```python
from build123d import *

# Parameters (mm, degrees)
BOSS_EXTRUDE1_DEPTH = 17.5
BOSS_EXTRUDE2_DEPTH = 5
CUT_EXTRUDE1_DEPTH  = 97.89865525603899
CUT_EXTRUDE2_DEPTH  = 97.89865525603899
CUT_EXTRUDE3_DEPTH  = 97.89865525603899
CUT_EXTRUDE4_DEPTH  = 97.89865525603899
CUT_EXTRUDE5_DEPTH  = 97.898655256039
HOLE1_D             = 3.4
HOLE2_D             = 8.4
HOLE3_D             = 4.4
HOLE4_D             = 23
HOLE5_D             = 8.4
HOLE6_D             = 4.4
FILLET1_R           = 8
CHAMFER1_SIZE       = 3.2892742843300167
CHAMFER1_SIZE2      = 5.503472902596259
CHAMFER2_SIZE       = 1.0000000000000073
CHAMFER3_SIZE       = 3.9999999999999973
CHAMFER4_SIZE       = 1.9999999999999982
CHAMFER5_SIZE       = 1.154784669
CHAMFER6_SIZE       = 0.9999999999999983
FILLET2_R           = 5
FILLET3_R           = 8.99999999999999
FILLET4_R           = 9.000000000000002


with BuildPart() as part:
    # Sketch1 → Boss-Extrude1 (new body)
    with BuildSketch(Plane(origin=(0, 0, 0), x_dir=(-6e-17, -1, 0), z_dir=(-1, 6e-17, 0))):
        with BuildLine():
            Line((11.200465877219063, 72.38053808131822), (-8.757531911002138, 37.812271894771776))
            ThreePointArc((-8.757531911002138, 37.812271894771776), (-19.5478712071735, 38.906001767514), (-24.988655696858714, 29.523809523809472))
            Line((-24.988655696858714, 29.523809523809472), (-23.581163303210467, 5.42e-15))
            Line((-23.581163303210467, 5.42e-15), (46.60534104687875, -6.94e-15))
            Line((46.60534104687875, -6.94e-15), (62.00126690227817, 42.299958639307405))
            Line((62.00126690227817, 42.299958639307405), (11.200465877219063, 72.38053808131822))
        make_face()
    extrude(amount=-BOSS_EXTRUDE1_DEPTH)

    # Sketch2 → Boss-Extrude2 (add)
    with BuildSketch(Plane(origin=(0, 0, 0), x_dir=(-6e-17, -1, 0), z_dir=(-1, 6e-17, 0))):
        with BuildLine():
            Line((-8.757531911002138, 37.812271894771776), (3.3020035333110394, 58.69999999999994))
            Line((3.3020035333110394, 58.69999999999994), (-12.000000000000004, 58.699999999999946))
            Line((-12.000000000000004, 58.699999999999946), (-12.000000000000004, 39.539392014169366))
            ThreePointArc((-12.000000000000004, 39.539392014169366), (-10.298772493194686, 38.826010419734104), (-8.757531911002138, 37.812271894771776))
        make_face()
    extrude(amount=-BOSS_EXTRUDE2_DEPTH)

    # Sketch3 → Cut-Extrude1 (cut, through all)
    with BuildSketch(Plane.ZY):
        with BuildLine():
            Line((18.94418997404675, -15.937202057164905), (20.43837116769735, -19.141483967443826))
            ThreePointArc((20.43837116769735, -19.141483967443826), (22.697545450618843, -19.96375616044696), (23.519817643621966, -17.70458187752546))
            Line((23.519817643621966, -17.70458187752546), (22.02563644997135, -14.500299967246516))
            ThreePointArc((22.02563644997135, -14.500299967246516), (19.766462167049855, -13.67802777424341), (18.94418997404675, -15.937202057164905))
        make_face()
    extrude(amount=-CUT_EXTRUDE1_DEPTH, mode=Mode.SUBTRACT)

    # Sketch4 → Cut-Extrude2 (cut, through all)
    with BuildSketch(Plane.ZY):
        with BuildLine():
            Line((48.89693341141304, -24.280652217339153), (45.692651501134065, -25.774833410989757))
            ThreePointArc((45.692651501134065, -25.774833410989757), (44.87037930813095, -28.034007693911235), (47.12955359105242, -28.85627988691438))
            Line((47.12955359105242, -28.85627988691438), (50.33383550133139, -27.362098693263775))
            ThreePointArc((50.33383550133139, -27.362098693263775), (51.156107694334516, -25.102924410342293), (48.89693341141304, -24.280652217339153))
        make_face()
    extrude(amount=-CUT_EXTRUDE2_DEPTH, mode=Mode.SUBTRACT)

    # Sketch5 → Cut-Extrude3 (cut, through all)
    with BuildSketch(Plane.ZY):
        with BuildLine():
            Line((35.97785558166356, -52.46601583434486), (37.47203677531419, -55.6702977446238))
            ThreePointArc((37.47203677531419, -55.6702977446238), (39.73121105823568, -56.4925699376269), (40.55348325123879, -54.233395654705404))
            Line((40.55348325123879, -54.233395654705404), (39.059302057588205, -51.02911374442645))
            ThreePointArc((39.059302057588205, -51.02911374442645), (36.80012777466672, -50.20684155142337), (35.97785558166356, -52.46601583434486))
        make_face()
    extrude(amount=-CUT_EXTRUDE3_DEPTH, mode=Mode.SUBTRACT)

    # Sketch6 → Cut-Extrude4 (cut, through all)
    with BuildSketch(Plane.ZY):
        with BuildLine():
            Line((10.600739813872503, -45.8899454945312), (13.805021724151473, -44.395764300880586))
            ThreePointArc((13.805021724151473, -44.395764300880586), (14.627293917154569, -42.136590017959094), (12.36811963423308, -41.314317824955985))
            Line((12.36811963423308, -41.314317824955985), (9.163837723954103, -42.8084990186066))
            ThreePointArc((9.163837723954103, -42.8084990186066), (8.341565530951023, -45.06767330152808), (10.600739813872503, -45.8899454945312))
        make_face()
    extrude(amount=-CUT_EXTRUDE4_DEPTH, mode=Mode.SUBTRACT)

    # Sketch7 → Cut-Extrude5 (cut, through all)
    with BuildSketch(Plane(origin=(17.5, -1.07e-15, 0), x_dir=(0, 0, -1), z_dir=(1, -6e-17, 0))):
        Polygon((-30.000000000000007, 8.000000000000005), (-30.000000000000007, -9.938112905604582), (-16.55393055212617, -9.938112905604578), (-10.000000000000002, -27.94488910624502), (-10.000000000000002, 8.000000000000005), align=None)
    extrude(amount=-CUT_EXTRUDE5_DEPTH, mode=Mode.SUBTRACT)

    # Hole1 (through all)
    with Locations(Plane(origin=(5, -3.1e-16, 0), x_dir=(0, 0, -1), z_dir=(1, -6e-17, 0))):
        with Locations((-50.7, 7)):
            Hole(HOLE1_D / 2)

    # Hole2 (through all)
    with Locations(Plane.ZY):
        with Locations((9, 15)):
            Hole(HOLE2_D / 2)

    # Hole3 (through all)
    with Locations(Plane.ZY):
        with Locations((40.5, -12.150669091)):
            Hole(HOLE3_D / 2)

    # Hole4 (through all)
    with Locations(Plane.ZY):
        with Locations((29.748836613, -35.085298856)):
            Hole(HOLE4_D / 2)

    # Hole5 (through all)
    with Locations(Plane.ZY):
        with Locations((60, -14.444863729)):
            Hole(HOLE5_D / 2)

    # Hole6 (through all)
    with Locations(Plane.ZY):
        with Locations((30, 15)):
            Hole(HOLE6_D / 2)

    # Fillet1
    fillet1_edges = [part.edges().sort_by_distance(p)[0] for p in [
        (11.25, 8.757531911002138, 37.812271894771776),
    ]]
    fillet(fillet1_edges, radius=FILLET1_R)

    # Chamfer1
    chamfer1_edges = [part.edges().sort_by_distance(p)[0] for p in [
        (8.75, -9.93811290560458, 16.55393055212617),
    ]]
    chamfer1_side = [part.faces().sort_by_distance(p)[0] for p in [
        (8.750000000000002, -18.941501005924803, 13.276965276063088),
    ]]
    chamfer(chamfer1_edges, length=CHAMFER1_SIZE, length2=CHAMFER1_SIZE2, reference=chamfer1_side[0])

    # Chamfer2
    chamfer2_edges = [part.edges().sort_by_distance(p)[0] for p in [
        (2.5, -3.3020035333110394, 58.69999999999994),
    ]]
    chamfer(chamfer2_edges, length=CHAMFER2_SIZE)

    # Chamfer3
    chamfer3_edges = [part.edges().sort_by_distance(p)[0] for p in [
        (2.500000000000001, 12.000000000000004, 58.699999999999946),
    ]]
    chamfer(chamfer3_edges, length=CHAMFER3_SIZE)

    # Chamfer4
    chamfer4_edges = [part.edges().sort_by_distance(p)[0] for p in [
        (8.75, 8.000000000000004, 10.000000000000002),
    ]]
    chamfer(chamfer4_edges, length=CHAMFER4_SIZE)

    # Chamfer5
    # the kernel refuses this chamfer: 1.339656624, 1.154784669 mm, written as the material it adds along each edge
    with BuildSketch(Plane(origin=(5.000000000000001, 12.000000000000004, 39.790087105703904), x_dir=(0, 0, 1), z_dir=(-1, 6e-17, 0))) as chamfer5_piece_1:
        with BuildLine():
            Line((CHAMFER5_SIZE, 0), (0.05834718904861802, 1.2292620817061763))
            ThreePointArc((0.05834718904861802, 1.2292620817061763), (0.00643151248669227, 0.6348707855031801), (0, 0))
            Line((0, 0), (CHAMFER5_SIZE, 0))
        make_face()
    extrude(amount=5)

    # Chamfer6
    chamfer6_edges = [part.edges().sort_by_distance(p)[0] for p in [
        (5.000000000000001, 0.7531265976075634, 51.67630858194548),
        (5, 8.674926913627807, 40.6231092014468),
    ]]
    chamfer(chamfer6_edges, length=CHAMFER6_SIZE)

    # Fillet2
    fillet2_edges = [part.edges().sort_by_distance(p)[0] for p in [
        (8.749999999999996, -62.00126690227817, 42.299958639307405),
    ]]
    fillet(fillet2_edges, radius=FILLET2_R)

    # Fillet3
    fillet3_edges = [part.edges().sort_by_distance(p)[0] for p in [
        (8.75, -11.200465877219063, 72.38053808131822),
    ]]
    fillet(fillet3_edges, radius=FILLET3_R)

    # Fillet4
    fillet4_edges = [part.edges().sort_by_distance(p)[0] for p in [
        (8.750000000000002, 23.581163303210467, 5.42e-15),
    ]]
    fillet(fillet4_edges, radius=FILLET4_R)


solid = part.part
```
Here's how the part is built. I have some questions about the finished solid (model axes, mm). A direction names the side the tool comes from. Coordinates: 2 decimals unless noted, no trailing zeros. Order: outer loops, then holes, each group sorted by start corner. A loop starts at its lowest first (then second) coordinate and runs counter-clockwise, first axis right, second up. Notation, with made-up numbers: (75.5, 73) -> (128.5, 73) arc R9 ccw to (128.5, 80) -> close; hole circle Ø11 at (48.5, -2). An arc over 180 degrees is marked (long way). Return JSON: item names as keys, results as strings.
1) If we section it at A-A on y = -38.5: List the corners of the cut face in (x, z) for me.
Conclusion:
{"outline": "(0, 0) -> (17.5, 0) -> (17.5, 18.77) -> (0, 18.77) -> close; (0, 40.73) -> (17.5, 40.73) -> (17.5, 56.22) -> (0, 56.22) -> close"}
2) On a 3-axis mill with a long thin cutter (end or side, diameter ignored), from which of +Z, -Z, +X, -X, +Y, -Y can I reach the whole of each face in a straight line? I mean faces 1 (the flat face through (5, 5, 52)), 2 (the flat face through (2, 12, 48)), 3 (the flat face through (8.628, -25.017, 47.317)). Say none if no direction works.
Conclusion:
{"face 1": "+Z, +X, +Y", "face 2": "+Z, +X, -X, +Y", "face 3": "+X, -X"}
3) If we section it at C-C on x = 10: State how many separate pieces and enclosed holes the cut face has, plus the area to 3 significant figures.
Conclusion:
{"separate pieces": "1", "enclosed holes": "10", "area": "3,200 mm²"}
4) Thinking about a two-plate mould opening in Z: for faces 4 (the cylindrical face through (8.87, 21.14, 2.42)), 5 (the cylindrical face through (8.627, -56.508, 39.697)), 6 (the flat face through (8.627, -39.007, 55.916)), which applies, +Z half, -Z half, draft (parallel to the pull), parting line (faces both ways), or undercut?
Conclusion:
{"face 4": "-Z half", "face 5": "undercut", "face 6": "+Z half"}
5) I'm going to push flat-ended pins straight in: P1, Ø8, axis at x = 12, z = 19.5, coming from the -Y side; P2, Ø1.5, axis at x = 2.5, y = 1.5, coming from the +Z side; P3, Ø1.5, axis at x = 3.5, z = 49.5, coming from the +Y side; P4, Ø7.5, axis at y = -14.44, z = 60, coming from the -X side. Where does each tip first touch, or does it pass through?
Conclusion:
{"P1": "stops at y = -55.16", "P2": "stops at z = 58.7", "P3": "stops at y = 12", "P4": "passes through"}
6) If I drill on probe 1 along Y at (x, z) = (3.25, 19.5); probe 2 along Y at (x, z) = (13.25, 9); probe 3 along Y at (x, z) = (2, 50), over which ranges is the centre line in solid material (lowest first)?
Conclusion:
{"probe 1": "y = -53.7 to -40.3, -29.87 to -17.13, -13.83 to -11.13, 8 to 24.51", "probe 2": "y = -49.88 to -45.8, -42.9 to 10.8, 19.2 to 24.01", "probe 3": "y = -49 to -27.52, -24.17 to 5.45, 8.55 to 12"}
7) If we section it at B-B on z = 34.5: List the corners of the cut face in (x, y) for me.
Conclusion:
{"outline": "(0, -59.16) -> (17.5, -59.16) -> (17.5, -45.56) -> (0, -45.56) -> close; (0, -24.61) -> (17.5, -24.61) -> (17.5, 23.93) -> (0, 23.93) -> close"}
